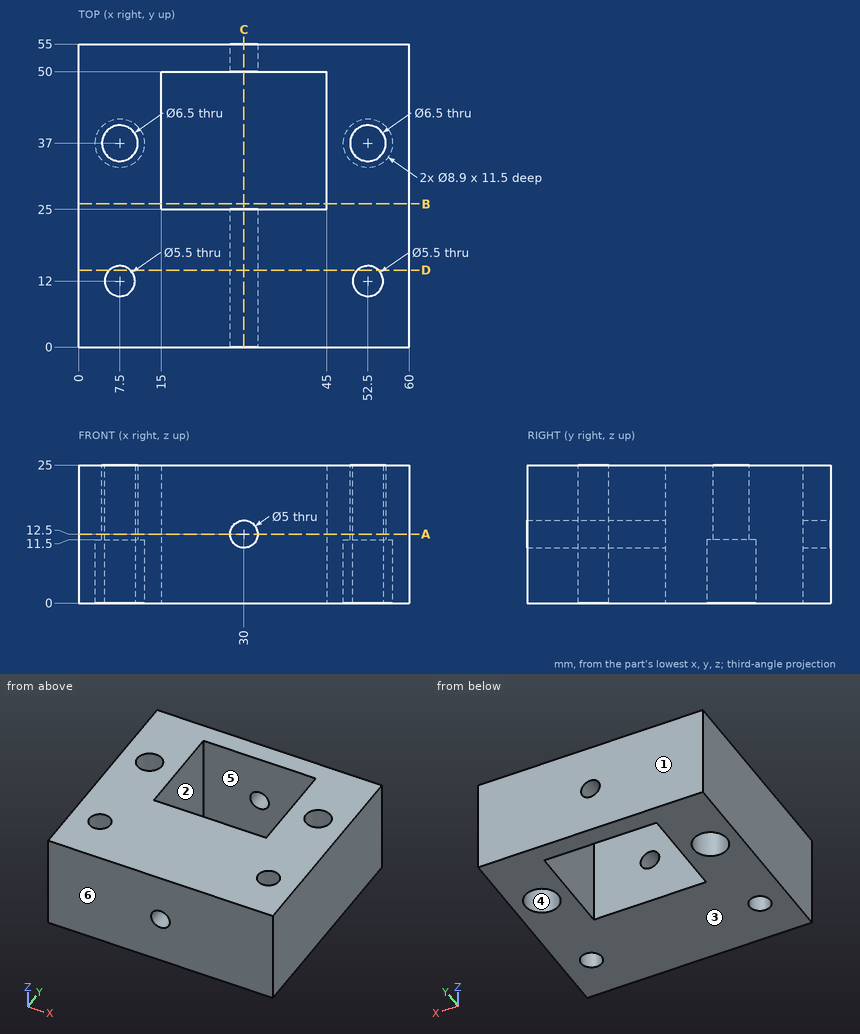
The drawing under review shows one solid part. Ordinate dimensions are in mm from its lowest x, y, z. A direction names the side the tool comes from. Give positions to 0.01 mm unless a question says otherwise; leave off trailing zeros. Write each loop counter-clockwise with the first axis right and the second up, starting at its lowest first coordinate (ties: lowest second). Pieces come first, ordered by that corner, then holes.
1. For P1, Ø3, axis at x = 30, z = 12.5, coming from the -Y side; P2, Ø4.5, axis at x = 6.5, y = 38, coming from the -Z side, all flat-tipped, find the tip position at first contact; note any pin that passes through.
2. Add section B-B, the plane y = 26. Write out the cut boundary in (x, z).
3. Wall thickness on L1, parallel to Y at x = 52.5, z = 6.25; L2, parallel to Y at x = 52.5, z = 15.25; L3, parallel to X at y = 38, z = 12.25: over which ranges is each line inside the solid? List them lowest first.
4. Add section D-D, the plane y = 14. Write out the cut boundary in (x, z).
5. Draft analysis for pull direction Y (two halves, no side actions). For the marked faces 1, 2 and 3, state which applies: +Y half, -Y half, draft (parallel to the pull), parting line (faces both ways), or undercut.
6. Add section A-A, the plane z = 12.5. Write out the cut boundary in (x, y), plus the area to 3 significant figures.
7. Add section C-C, the plane x = 30. Write out the cut boundary in (y, z), plus the area to 3 significant figures.
8. Tool access review of the marked faces 4, 5 and 6: name each direction out of +Z, -Z, +X, -X, +Y, -Y from which nothing blocks a thin tool from reaching the whole face with its end or side.
Worked answers:
1. P1: passes through
1. P2: stops at z = 11.5
2. outline: (0, 0) - (15, 0) - (15, 25) - (0, 25) - close; (45, 0) - (60, 0) - (60, 25) - (45, 25) - close
3. L1: y = 0 to 9.25, 14.75 to 32.55, 41.45 to 55
3. L2: y = 0 to 9.25, 14.75 to 33.75, 40.25 to 55
3. L3: x = 0 to 4.41, 10.59 to 15, 45 to 49.41, 55.59 to 60
4. outline: (0, 0) - (5.61, 0) - (5.61, 25) - (0, 25) - close; (9.39, 0) - (50.61, 0) - (50.61, 25) - (9.39, 25) - close; (54.39, 0) - (60, 0) - (60, 25) - (54.39, 25) - close; hole circle Ø5 at (30, 12.5)
5. face 1: +Y half
5. face 2: undercut
5. face 3: draft
6. outline: (0, 0) - (27.5, 0) - (27.5, 25) - (15, 25) - (15, 50) - (27.5, 50) - (27.5, 55) - (0, 55) - close; (32.5, 0) - (60, 0) - (60, 55) - (32.5, 55) - (32.5, 50) - (45, 50) - (45, 25) - (32.5, 25) - close; hole circle Ø6.5 at (7.5, 37); hole circle Ø5.5 at (7.5, 12); hole circle Ø6.5 at (52.5, 37); hole circle Ø5.5 at (52.5, 12)
6. area: 2,290 mm2
7. outline: (0, 0) - (25, 0) - (25, 10) - (0, 10) - close; (0, 15) - (25, 15) - (25, 25) - (0, 25) - close; (50, 0) - (55, 0) - (55, 10) - (50, 10) - close; (50, 15) - (55, 15) - (55, 25) - (50, 25) - close
7. area: 600 mm2
8. face 4: -Z
8. face 5: +Z, -Z
8. face 6: +Z, -Z, +X, -X, -Y
